Solid Edge part; units mm, degrees
sketch "Sketch1" plane through (0, 0, 0) normal (0, 0, 1) x (1, 0, 0)
  circle A0 centre (0, 0) radius 9.75
extrude "Protrusion1" add sketch "Sketch1" along normal blind 2
sketch "Sketch2" plane through (0, 0, 0) normal (0, 0, -1) x (1, 0, 0)
  circle A0 centre (0, 0) radius 6.5
extrude "Protrusion2" add sketch "Sketch2" along normal blind 22
sketch "Sketch3" plane through (0, 0, -22) normal (0, 0, -1) x (1, 0, 0)
  line L0 (-3.5, 3.5707) -> (-3.5, -3.5707)
  arc A0 (-3.5, 3.5707) -> (-3.5, -3.5707) centre (0, 0) cw
extrude "Protrusion3" add sketch "Sketch3" along normal blind 8
sketch "Sketch4" plane through (0, 0, 2) normal (0, 0, 1) x (1, 0, 0)
  line L0 (-3.4699, 3.6) -> (3.4699, 3.6)
  arc A0 (3.4699, 3.6) -> (3.4699, -3.6) centre (0, 0) cw
  line L1 (3.4699, -3.6) -> (-3.4699, -3.6)
  arc A1 (-3.4699, -3.6) -> (-3.4699, 3.6) centre (0, 0) cw
extrude "Cutout1" cut sketch "Sketch4" against normal blind 14
properties part number "SHAFT1" material "4140 Steel"
Work out the finished part from the listing and answer in its coordinate system (mm). A direction names the side the tool comes from. Coordinates: 2 decimals unless noted, no trailing zeros. Order: outer loops, then holes, each group sorted by start corner. A loop starts at its lowest first (then second) coordinate and runs counter-clockwise, first axis right, second up. Notation, with made-up numbers: (10.5, 29.5) - (29.5, 29.5) arc R18 cw to (29.5, 57.5) - close; hole circle Ø1 at (70.25, 72). An arc over 180 degrees is marked (long way). Put each result on its own line as item: value. Start each with the question number.
1) For a pull along Y with two mould halves and no side action, classify faces 1 (the cylindrical face through (-1.269, -9.667, 0.986)), 2 (the cylindrical face through (-5, 0, -5)), 3 (the flat face through (2, -6.4, 0)) as released by +Y, released by -Y, zero draft, split by the parting line, or undercut.
2) Find section A-A (z = -10.5). Give the vertices of the cut face in (x, y).
3) For faces 4 (the flat face through (0, 3.6, -5)), 5 (the cylindrical face through (-5.158, -3.955, -10.846)), 6 (the flat face through (-3.5, 0, -26)), determine the directions among +Z, -Z, +X, -X, +Y, -Y from which every point of the face is accessible in a straight line to the end or side of a thin tool.
4) Flat-ended cylindrical pins translate along their axes: pin 1 (5.5 mm diameter, centred on y = -1.5, z = -25, fed in from -X); pin 2 (1.5 mm diameter, centred on x = 6, y = 4, fed in from -Z); pin 3 (5.5 mm diameter, centred on x = 0, z = -5, fed in from -Y). Find the tip coordinate at first contact, or state that the pin passes through.
5) Find section B-B (y = 0). Give the vertices of the cut face in (x, z), plus the area to 3 significant figures.
6) Find the intervals of material crossed by line 1 (Z direction, x = -4.25, y = -2.5); line 2 (Z direction, x = 5.75, y = -0.75); line 3 (Y direction, x = -5.5, z = -13), in increasing order. Write a range as from..to.
7) Find section D-D (z = -16). Give the vertices of the cut face in (x, y), plus the area to 3 significant figures.
8) Find section C-C (x = 0). Give the vertices of the cut face in (y, z), plus the area to 3 significant figures.
Results list:
1. face 1: split by the parting line
1. face 2: undercut
1. face 3: zero draft
2. outline: circle Ø13 at (0, 0); hole (-3.47, -3.6) - (3.47, -3.6) arc R5 ccw to (3.47, 3.6) - (-3.47, 3.6) arc R5 ccw to start
3. face 4: +Z
3. face 5: -Z
3. face 6: -Z, -X, +Y, -Y
4. pin 1: stops at x = -3.5
4. pin 2: stops at z = -22
4. pin 3: stops at y = -6.5
5. outline: (-9.75, 0) - (-6.5, 0) - (-6.5, -22) - (-3.5, -22) - (-3.5, -30) - (5, -30) - (5, -22) - (6.5, -22) - (6.5, 0) - (9.75, 0) - (9.75, 2) - (5, 2) - (5, -12) - (-5, -12) - (-5, 2) - (-9.75, 2) - close
5. area: 253 mm^2
6. line 1: z = -22..-12
6. line 2: z = -22..2
6. line 3: y = -3.46..3.46
7. outline: circle Ø13 at (0, 0)
7. area: 133 mm^2
8. outline: (-9.75, 0) - (-6.5, 0) - (-6.5, -22) - (-5, -22) - (-5, -30) - (5, -30) - (5, -22) - (6.5, -22) - (6.5, 0) - (9.75, 0) - (9.75, 2) - (3.6, 2) - (3.6, -12) - (-3.6, -12) - (-3.6, 2) - (-9.75, 2) - close
8. area: 304 mm^2
